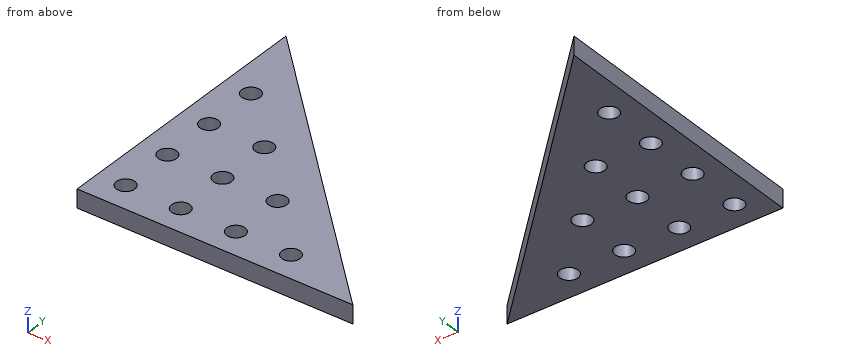
```python
from build123d import *

# Parameters (mm, degrees)
MODEL_R                 = 1.5
SALIENTE_EXTRUIR1_DEPTH = 3


with BuildPart() as part:
    # Model → Saliente-Extruir1 (new body)
    with BuildSketch(Plane.XY):
        Polygon((-105.943383637, 105.556539338), (-105.943383637, 60.556539338), (-60.943383637, 60.556539338), align=None)
        with Locations((-101.443383637, 92.056539338)):
            Circle(MODEL_R, mode=Mode.SUBTRACT)
        with Locations((-101.443383637, 83.056539338)):
            Circle(MODEL_R, mode=Mode.SUBTRACT)
        with Locations((-92.443383637, 83.056539338)):
            Circle(MODEL_R, mode=Mode.SUBTRACT)
        with Locations((-101.443383637, 74.056539338)):
            Circle(MODEL_R, mode=Mode.SUBTRACT)
        with Locations((-92.443383637, 74.056539338)):
            Circle(MODEL_R, mode=Mode.SUBTRACT)
        with Locations((-83.443383637, 74.056539338)):
            Circle(MODEL_R, mode=Mode.SUBTRACT)
        with Locations((-101.443383637, 65.056539338)):
            Circle(MODEL_R, mode=Mode.SUBTRACT)
        with Locations((-92.443383637, 65.056539338)):
            Circle(MODEL_R, mode=Mode.SUBTRACT)
        with Locations((-83.443383637, 65.056539338)):
            Circle(MODEL_R, mode=Mode.SUBTRACT)
        with Locations((-74.443383637, 65.056539338)):
            Circle(MODEL_R, mode=Mode.SUBTRACT)
    extrude(amount=SALIENTE_EXTRUIR1_DEPTH)


solid = part.part
```
Here's how the part is built. I have some questions about the finished solid (model axes, mm). Round coordinates to 2 decimals unless told otherwise and drop trailing zeros. Loops run counter-clockwise (first coordinate to the right, second up) from the corner with the lowest first, then second, coordinate; pieces in that order, holes last. Notation, with made-up numbers: (-37.5, -13.5) -> (-6.5, -13.5) arc R12 cw to (-6.5, -3.5) -> close; hole circle Ø6 at (-30.75, 65). An arc over 180 degrees is marked (long way). Answer as CSV lines item,"result". Start each with the question number.
1. Imagine slicing it at B-B on x = -74. Write out the boundary of the cut face in (y, z), plus the area to 3 significant figures.
2. Imagine slicing it at D-D on y = 63. Write out the boundary of the cut face in (x, z), plus the area to 3 significant figures.
3. Imagine slicing it at C-C on z = 1.4. State how many separate pieces and enclosed holes the cut face has, plus the area to 3 significant figures.
4. I need wall thicknesses on probe 1 along X at (y, z) = (73.5, 2.7); probe 2 along Y at (x, z) = (-91.5, 2.55); probe 3 along X at (y, z) = (83, 0.5). Which ranges of each line are inside material? Lowest first, please. Write a range as from..to.
5. Imagine slicing it at A-A on x = -84. Write out the boundary of the cut face in (y, z), plus the area to 3 significant figures.
6. I'm going to push flat-ended pins straight in: P1, Ø2.5, axis at x = -83.44, y = 65.06, coming from the +Z side; P2, Ø4, axis at x = -92.44, y = 83.06, coming from the -Z side; P3, Ø1, axis at x = -85, z = 0.5, coming from the +Y side. Where does each tip first touch, or does it pass through?
Solution:
1,outline,"(60.56, 0) -> (63.62, 0) -> (63.62, 3) -> (60.56, 3) -> close; (66.49, 0) -> (73.61, 0) -> (73.61, 3) -> (66.49, 3) -> close"
1,area,"30.6 mm²"
2,outline,"(-105.94, 0) -> (-63.39, 0) -> (-63.39, 3) -> (-105.94, 3) -> close"
2,area,"128 mm²"
3,separate pieces,"1"
3,enclosed holes,"10"
3,area,"942 mm²"
4,probe 1,"-105.94..-102.84, -100.05..-93.84, -91.05..-84.84, -82.05..-73.89"
4,probe 2,"60.56..63.89, 66.22..72.89, 75.22..81.89, 84.22..91.11"
4,probe 3,"-105.94..-102.94, -99.94..-93.94, -90.94..-83.39"
5,outline,"(60.56, 0) -> (63.66, 0) -> (63.66, 3) -> (60.56, 3) -> close; (66.45, 0) -> (72.66, 0) -> (72.66, 3) -> (66.45, 3) -> close; (75.45, 0) -> (83.61, 0) -> (83.61, 3) -> (75.45, 3) -> close"
5,area,"52.5 mm²"
6,P1,"through"
6,P2,"z = 0"
6,P3,"y = 85.11"
